Can you work these out from the model? Positions are in its coordinate system, mm. A direction names the side the tool comes from. Give positions to 0.01 mm unless a question says otherwise; leave off trailing zeros. Write each loop counter-clockwise with the first axis right and the second up, starting at its lowest first coordinate (ties: lowest second). Pieces come first, ordered by that corner, then holes. Notation, with made-up numbers: (75, 23) - (86, 23) arc R17 ccw to (86, 30) - close; hole circle Ø9 at (-4.75, 87.5). An arc over 180 degrees is marked (long way). Return JSON: item names as keys, results as strings. Group by question number.
Autodesk Inventor part; units mm, degrees
ref_plane "b1_XY" through (0, 7.8994, 0) normal (1, 0, 0) x (0, 0, -1)
ref_plane "b1_YZ" through (0, 7.8994, 0) normal (0, 0, -1) x (0, 1, 0)
ref_plane "b1_ZX" through (0, 7.8994, 0) normal (0, 1, 0) x (1, 0, 0)
sketch "Sketch_1" plane through (0, 0, 0) normal (0, 0, 1) x (1, 0, 0)
  line L0 (14.0462, 0) -> (0, 0)
  line L1 (0, 0) -> (0, 10.8585)
  line L2 (0, 10.8585) -> (14.0462, 10.8585)
  line L3 (14.0462, 10.8585) -> (14.0462, 0)
  line L4 (14.0462, 0) -> (0, 0)
revolve "Revolution1" add sketch "Sketch_1" angle 360 about axis through (14.0462, 0, 0) along (1, 0, 0)
sketch "Sketch_2" plane through (0, 0, 0) normal (0, 0, 1) x (1, 0, 0)
  line L0 (0, 0) -> (-15.9766, 0)
  line L1 (-15.9766, 0) -> (-15.9766, 7.098)
  line L2 (-15.9766, 7.098) -> (-15.1371, 7.9375)
  line L3 (-15.1371, 7.9375) -> (0, 7.9375)
  line L4 (0, 7.9375) -> (0, 0)
  line L5 (0, 0) -> (-15.9766, 0)
revolve "Revolution2" add sketch "Sketch_2" angle 360 about axis through (0, 0, 0) along (1, 0, 0)
thread "Thread1"
sketch "Sketch_6" plane through (0, 0, 0) normal (0, 0, 1) x (1, 0, 0)
  line L0 (23.6982, 0) -> (14.0462, 0)
  line L1 (14.0462, 0) -> (14.0462, 10.3505)
  line L2 (14.0462, 10.3505) -> (18.2372, 10.3505)
  line L3 (18.2372, 10.3505) -> (18.2372, 8.9027)
  line L4 (18.2372, 8.9027) -> (19.1516, 8.9027)
  line L5 (19.1516, 8.9027) -> (19.8755, 9.6266)
  line L6 (19.8755, 9.6266) -> (22.9362, 9.6266)
  line L7 (22.9362, 9.6266) -> (23.6982, 8.8646)
  line L8 (23.6982, 8.8646) -> (23.6982, 0)
  line L9 (23.6982, 0) -> (14.0462, 0)
revolve "Revolution3" add sketch "Sketch_6" angle 360 about axis through (23.6982, 0, 0) along (1, 0, 0)
sketch "Sketch_8" plane through (7.0612, 0, 0) normal (0, 0, 1) x (0, -1, 0)
  line L0 (0, 0) -> (-11.7085, 0)
  line L1 (-11.7085, 0) -> (-11.7085, 6.4547)
  line L2 (-11.7085, 6.4547) -> (-10.0692, 4.8153)
  line L3 (-10.0692, 4.8153) -> (0, 4.501)
  line L4 (0, 4.501) -> (0, 0)
  line L5 (0, 0) -> (-11.7085, 0)
revolve "Revolution4" cut sketch "Sketch_8" angle 360 about axis through (7.0612, 0, 0) along (0, -1, 0)
sketch "Sketch_29" plane through (0, 0, 0) normal (0, 0, 1) x (1, 0, 0)
  line L0 (0, 0) -> (-5.2578, 0)
  line L1 (-5.2578, 9.8994) -> (-5.2578, 7.9375)
  line L2 (-5.2578, 7.9375) -> (-4.3634, 7.0431)
  arc A0 (-4.3634, 7.0431) -> (-3.8246, 6.8199) centre (-3.8246, 7.5819) ccw
  line L3 (-3.8246, 6.8199) -> (-2.7567, 6.8199)
  arc A1 (-2.7567, 6.8199) -> (-2.0828, 7.2263) centre (-2.7567, 7.5819) ccw
  line L4 (-2.0828, 7.2263) -> (-2.0828, 7.8994)
  line L5 (-2.0828, 7.8994) -> (0, 7.8994)
  line L6 (0, 7.8994) -> (0, 9.8994)
  line L7 (0, 9.8994) -> (-5.2578, 9.8994)
revolve "Revolution5" cut sketch "Sketch_29" angle 360 about axis through (0, 0, 0) along (1, 0, 0)
sketch "Sketch_38" plane through (-0.2032, 0, 0) normal (1, 0, 0) x (0, 0, -1)
  line L0 (-10.8585, -10.8585) -> (10.8585, -10.8585)
  line L1 (10.8585, -10.8585) -> (10.8585, 10.8585)
  line L2 (10.8585, 10.8585) -> (-10.8585, 10.8585)
  line L3 (-10.8585, 10.8585) -> (-10.8585, -10.8585)
  line L4 (-4.699, -8.7312) -> (4.699, -8.7312)
  line L5 (4.699, -8.7312) -> (4.699, 8.7312)
  line L6 (4.699, 8.7312) -> (-4.699, 8.7312)
  line L7 (-4.699, 8.7312) -> (-4.699, -8.7312)
extrude "Extrusion1" cut sketch "Sketch_38" against normal blind 15.9766
sketch "Sketch_36" plane through (0, 0, 0) normal (0, 1, 0) x (-1, 0, 0)
  line L0 (8.9408, 4.699) -> (8.9408, -4.699)
  line L1 (8.9408, -4.699) -> (5.1079, -4.699)
  line L2 (5.1079, -4.699) -> (5.7467, -4.0602)
  line L3 (5.7467, -4.0602) -> (5.7467, 4.0602)
  line L4 (5.7467, 4.0602) -> (5.1079, 4.699)
  line L5 (5.1079, 4.699) -> (8.9408, 4.699)
  line L6 (8.9408, 4.699) -> (8.9408, -4.699)
revolve "Revolution6" cut sketch "Sketch_36" angle 360 about axis through (-8.9408, 0, 4.699) along (0, 0, 1)
ref_plane "b1_XY" through (0, 7.8994, 0) normal (1, 0, 0) x (0, 0, -1)
ref_plane "b1_YZ" through (0, 7.8994, 0) normal (0, 0, -1) x (0, 1, 0)
ref_plane "b1_ZX" through (0, 7.8994, 0) normal (0, 1, 0) x (1, 0, 0)
ref_plane "b2_XY" through (0, -7.8994, 0) normal (1, 0, 0) x (0, 0, -1)
ref_plane "b2_YZ" through (0, -7.8994, 0) normal (0, 0, -1) x (0, 1, 0)
ref_plane "b2_ZX" through (0, -7.8994, 0) normal (0, 1, 0) x (1, 0, 0)
ref_plane "cl1_XY" through (0, 0, 0) normal (0, 0, 1) x (1, 0, 0)
ref_plane "cl1_YZ" through (0, 0, 0) normal (1, 0, 0) x (0, 1, 0)
ref_plane "cl1_ZX" through (0, 0, 0) normal (0, 1, 0) x (0, 0, 1)
ref_plane "cl2_XY" through (-2.0828, 0, 0) normal (0, 0, 1) x (1, 0, 0)
ref_plane "cl2_YZ" through (-2.0828, 0, 0) normal (1, 0, 0) x (0, 1, 0)
ref_plane "cl2_ZX" through (-2.0828, 0, 0) normal (0, 1, 0) x (0, 0, 1)
ref_plane "ecut1_XY" through (-0.2032, 0, 4.699) normal (1, 0, 0) x (0, 0, -1)
ref_plane "ecut1_YZ" through (-0.2032, 0, 4.699) normal (0, 0, -1) x (0, 1, 0)
ref_plane "ecut1_ZX" through (-0.2032, 0, 4.699) normal (0, 1, 0) x (1, 0, 0)
ref_plane "ecut2_XY" through (-0.2032, 0, -4.699) normal (1, 0, 0) x (0, 0, -1)
ref_plane "ecut2_YZ" through (-0.2032, 0, -4.699) normal (0, 0, -1) x (0, 1, 0)
ref_plane "ecut2_ZX" through (-0.2032, 0, -4.699) normal (0, 1, 0) x (1, 0, 0)
ref_plane "ee_XY" through (7.0612, 10.8585, 0) normal (1, 0, 0) x (0, -1, 0)
ref_plane "ee_YZ" through (7.0612, 10.8585, 0) normal (0, -1, 0) x (0, 0, -1)
ref_plane "ee_ZX" through (7.0612, 10.8585, 0) normal (0, 0, -1) x (1, 0, 0)
ref_plane "od1_XY" through (0, 0, 10.8585) normal (1, 0, 0) x (0, 0, -1)
ref_plane "od1_YZ" through (0, 0, 10.8585) normal (0, 0, -1) x (0, 1, 0)
ref_plane "od1_ZX" through (0, 0, 10.8585) normal (0, 1, 0) x (1, 0, 0)
ref_plane "od2_XY" through (0, 0, -10.8585) normal (1, 0, 0) x (0, 0, -1)
ref_plane "od2_YZ" through (0, 0, -10.8585) normal (0, 0, -1) x (0, 1, 0)
ref_plane "od2_ZX" through (0, 0, -10.8585) normal (0, 1, 0) x (1, 0, 0)
ref_plane "od3_XY" through (0, 10.8585, 0) normal (1, 0, 0) x (0, 0, -1)
ref_plane "od3_YZ" through (0, 10.8585, 0) normal (0, 0, -1) x (0, 1, 0)
ref_plane "od3_ZX" through (0, 10.8585, 0) normal (0, 1, 0) x (1, 0, 0)
ref_plane "od4_XY" through (0, -10.8585, 0) normal (1, 0, 0) x (0, 0, -1)
ref_plane "od4_YZ" through (0, -10.8585, 0) normal (0, 0, -1) x (0, 1, 0)
ref_plane "od4_ZX" through (0, -10.8585, 0) normal (0, 1, 0) x (1, 0, 0)
ref_plane "to_body_XY" through (18.2372, 0, 0) normal (1, 0, 0) x (0, 0, -1)
ref_plane "to_body_YZ" through (18.2372, 0, 0) normal (0, 0, -1) x (0, 1, 0)
ref_plane "to_body_ZX" through (18.2372, 0, 0) normal (0, 1, 0) x (1, 0, 0)
ref_plane "to_dummy_XY" through (0, 0, 0) normal (1, 0, 0) x (0, 0, -1)
ref_plane "to_dummy_YZ" through (0, 0, 0) normal (0, 0, -1) x (0, 1, 0)
ref_plane "to_dummy_ZX" through (0, 0, 0) normal (0, 1, 0) x (1, 0, 0)
ref_plane "to_nut_XY" through (-15.9766, 0, 0) normal (1, 0, 0) x (0, 0, -1)
ref_plane "to_nut_YZ" through (-15.9766, 0, 0) normal (0, 0, -1) x (0, 1, 0)
ref_plane "to_nut_ZX" through (-15.9766, 0, 0) normal (0, 1, 0) x (1, 0, 0)
ref_plane "to_pin_XY" through (-8.9408, 0, 0) normal (0, 0, 1) x (1, 0, 0)
ref_plane "to_pin_YZ" through (-8.9408, 0, 0) normal (1, 0, 0) x (0, 1, 0)
ref_plane "to_pin_ZX" through (-8.9408, 0, 0) normal (0, 1, 0) x (0, 0, 1)
ref_plane "to_stroke_adjuster_XY" through (23.6982, 0, 0) normal (1, 0, 0) x (0, 0, -1)
ref_plane "to_stroke_adjuster_YZ" through (23.6982, 0, 0) normal (0, 0, -1) x (0, 1, 0)
ref_plane "to_stroke_adjuster_ZX" through (23.6982, 0, 0) normal (0, 1, 0) x (1, 0, 0)
ref_plane "z1_XY" through (-8.9408, 3.194, 0) normal (0, 0, 1) x (1, 0, 0)
ref_plane "z1_YZ" through (-8.9408, 3.194, 0) normal (1, 0, 0) x (0, 1, 0)
ref_plane "z1_ZX" through (-8.9408, 3.194, 0) normal (0, 1, 0) x (0, 0, 1)
ref_plane "z2_XY" through (-8.9408, -3.194, 0) normal (0, 0, 1) x (1, 0, 0)
ref_plane "z2_YZ" through (-8.9408, -3.194, 0) normal (1, 0, 0) x (0, 1, 0)
ref_plane "z2_ZX" through (-8.9408, -3.194, 0) normal (0, 1, 0) x (0, 0, 1)
properties part number "0.75DXP-C_SRS10"
1) We'd pull the mould along Y, two halves only. Please class faces 1 (the face through (-0.203, 0, -6)), 2 (the face through (11.506, 5.105, -1.4)), 3 (the face through (-5.894, 0.959, 0.057)): pulls with the +Y half, pulls with the -Y half, needs draft (parallel to the pull), parting line crosses it, or undercut.
2) I need wall thicknesses on line 1 along Z through (x, y) = (-1.5, -3); line 2 along X through (y, z) = (-8.25, -1); line 3 along Z through (x, y) = (-4, 5.5). Which ranges of each line are inside material? Lowest first, please.
3) Will these pins go through, and if not, where does the flat tip stop? pin 1 Ø1.5 at (x, y) = (18.5, 0) entering from -Z; pin 2 Ø4 at (x, y) = (-5.5, 3) entering from -Z; pin 3 Ø4 at (x, z) = (-6.5, 1) entering from +Y; pin 4 Ø3 at (x, y) = (14, 1) entering from +Z.
4) On a 3-axis mill with a long thin cutter (end or side, diameter ignored), from which of +Z, -Z, +X, -X, +Y, -Y can I reach the whole of each face in a straight line? I mean faces 4 (the face through (-10.128, 7.937, -0.07)), 5 (the face through (-6, 3, 4.699)), 6 (the face through (-2.083, -7.4, 0.7)), 7 (the face through (-10.128, -7.937, 0.07)). Say none if no direction works.
5) Imagine slicing it at A-A, the plane x = 20.5. Write out the boundary of the cut face in (y, z), and give its area (3 significant figures).
Resolved:
{
 "1": {"face 1": "needs draft", "face 2": "pulls with the +Y half", "face 3": "undercut"},
 "2": {"line 1": "-4.7 to 4.7", "line 2": "0 to 23.7", "line 3": "-4.07 to 4.07"},
 "3": {"pin 1": "z = -10.35", "pin 2": "z = -4.7", "pin 3": "y = 7.94", "pin 4": "z = 10.86"},
 "4": {"face 4": "-X, +Y", "face 5": "+Z, -X, +Y, -Y", "face 6": "-Y", "face 7": "-X, -Y"},
 "5": {"outline": "circle Ø19.25 at (0, 0)", "area": "291 mm^2"}
}
